Geometry check sheet. Reference: the model listing, model coordinates, mm. A direction names the side the tool comes from. Coordinates: 2 decimals unless noted, no trailing zeros. Loops run counter-clockwise (first coordinate to the right, second up) from the corner with the lowest first, then second, coordinate; pieces in that order, holes last. Notation, with made-up numbers: (24.25, 34) - (56.25, 34) arc R20 cw to (56.25, 64) - close; hole circle Ø7 at (-20, 18.5). An arc over 180 degrees is marked (long way). Write item = value, one per line. Start each with the question number.
Solid Edge part; units mm, degrees
sketch "Sketch1" plane through (0, 0, 0) normal (0, -1, 0) x (1, 0, 0)
  line L0 (25, 0) -> (25, -9)
  arc A0 (25, -9) -> (31, -15) centre (31, -9) ccw
  line L1 (31, -15) -> (40, -15)
  arc A1 (46, -9) -> (40, -15) centre (40, -9) cw
  line L2 (46, 0) -> (46, -9)
  line L3 (56, 0) -> (46, 0)
  line L4 (56, -25) -> (56, 0)
  line L5 (-56, -25) -> (56, -25)
  line L6 (-56, 0) -> (-56, -25)
  line L7 (-46, 0) -> (-56, 0)
  line L8 (-46, -9) -> (-46, 0)
  arc A2 (-46, -9) -> (-40, -15) centre (-40, -9) ccw
  line L9 (-31, -15) -> (-40, -15)
  arc A3 (-25, -9) -> (-31, -15) centre (-31, -9) cw
  line L10 (-25, 0) -> (-25, -9)
  arc A4 (-25, 0) -> (25, 0) centre (0, 0) cw
  circle A5 centre (0, 0) radius 12.5
extrude "Protrusion1" add sketch "Sketch1" against normal blind 76
sketch "Sketch2" plane through (56, 38, -12.5) normal (1, 0, 0) x (0, 1, 0)
  line L0 (-28, -12.5) -> (-28, -22.5)
  line L1 (-28, -22.5) -> (-22, -22.5)
  line L2 (-22, -22.5) -> (-22, -12.5)
  line L3 (-22, -12.5) -> (-28, -12.5)
  line L4 (22, -12.5) -> (22, -22.5)
  line L5 (22, -22.5) -> (28, -22.5)
  line L6 (28, -22.5) -> (28, -12.5)
  line L7 (28, -12.5) -> (22, -12.5)
extrude "ExtrudedProtrusion_2" add sketch "Sketch2" against normal blind 112
(1) Sectioned sample at D-D on z = -5.5. Enter the section's corners in (x, y), plus the area to 3 significant figures.
(2) Sectioned sample at B-B on z = -29. Enter the section's corners in (x, y), plus the area to 3 significant figures.
(3) Tool access check on faces 4 (the face through (-25, 37, -4)), 5 (the face through (-1, 71, -25)), 6 (the face through (-51, 37, 0)), 7 (the face through (1, 10, -30)), 8 (the face through (-1, 38, -25)). Record the directions out of +Z, -Z, +X, -X, +Y, -Y that give a thin tool (end or side, any length) a straight path to the whole face; none if there is none.
(4) Sectioned sample at C-C on y = 64. Enter the section's corners in (x, z).
(5) Depth check by flat-ended pin: pin 1 (13 mm diameter, centred on x = 17, y = 28, fed in from -Z); pin 2 (7 mm diameter, centred on x = 35.5, y = 47, fed in from +Z); pin 3 (5 mm diameter, centred on x = 2.5, z = -30.5, fed in from +Y). Enter the tip coordinate at first touch or a pass-through.
(6) Scan lines: line 1 (Y direction, x = 19, z = -28); line 2 (Z direction, x = 0, y = 34.5); line 3 (X direction, y = 54.5, z = -3). Record each from-to range of solid material in increasing order.
(7) Sectioned sample at A-A on x = 0. Enter the section's corners in (y, z).
(8) Draft check along X on faces 1 (the face through (-44.289, 37.468, -13.196)), 2 (the face through (51, 37, 0)), 3 (the face through (-56, 37, -13)). Enter one of: pulls with the +X half, pulls with the -X half, needs draft (parallel to the pull), parting line crosses it, or undercut.
Working result:
q1.outline = (-56, 0) - (-46, 0) - (-46, 76) - (-56, 76) - close; (-25, 0) - (-11.22, 0) - (-11.22, 76) - (-25, 76) - close; (11.22, 0) - (25, 0) - (25, 76) - (11.22, 76) - close; (46, 0) - (56, 0) - (56, 76) - (46, 76) - close
q1.area = 3,610 mm2
q2.outline = (-56, 10) - (56, 10) - (56, 16) - (-56, 16) - close; (-56, 60) - (56, 60) - (56, 66) - (-56, 66) - close
q2.area = 1,340 mm2
q3.face_4 = +Z, +Y, -Y
q3.face_5 = -Z, +X, -X, +Y
q3.face_6 = +Z, -X, +Y, -Y
q3.face_7 = -Z, +X, -X, -Y
q3.face_8 = -Z, +X, -X
q4.outline = (-56, -35) - (56, -35) - (56, 0) - (46, 0) - (46, -9) arc R6 cw to (40, -15) - (31, -15) arc R6 cw to (25, -9) - (25, 0) arc R25 ccw to (-25, 0) - (-25, -9) arc R6 cw to (-31, -15) - (-40, -15) arc R6 cw to (-46, -9) - (-46, 0) - (-56, 0) - close; hole circle Ø25 at (0, 0)
q5.pin_1 = -25
q5.pin_2 = -15
q5.pin_3 = 66
q6.line_1 = 10 to 16, 60 to 66
q6.line_2 = -25 to -12.5, 12.5 to 25
q6.line_3 = -56 to -46, -25 to -12.13, 12.13 to 25, 46 to 56
q7.outline = (0, -25) - (10, -25) - (10, -35) - (16, -35) - (16, -25) - (60, -25) - (60, -35) - (66, -35) - (66, -25) - (76, -25) - (76, -12.5) - (0, -12.5) - close; (0, 12.5) - (76, 12.5) - (76, 25) - (0, 25) - close
q8.face_1 = undercut
q8.face_2 = needs draft
q8.face_3 = pulls with the -X half
